```python
from build123d import *

# Parameters (mm, degrees)
F0_W     = 19.05
F0_H     = 19.05
F1_DEPTH = 19.05


with BuildPart() as f1:
    # F0 (on Front) → F1 (new body)
    with BuildSketch(Plane.XZ):
        with Locations((-9.525, 9.525)):
            Rectangle(F0_W, F0_H)
        Polygon((0, 0), (-19.05, 0), (-38.1, 0), (-38.1, -19.05), (-19.05, -19.05), (-19.05, -38.1), (0, -38.1), (0, -19.05), (19.05, -19.05), (19.05, 0), align=None)
    extrude(amount=F1_DEPTH)


solid = f1.part
```
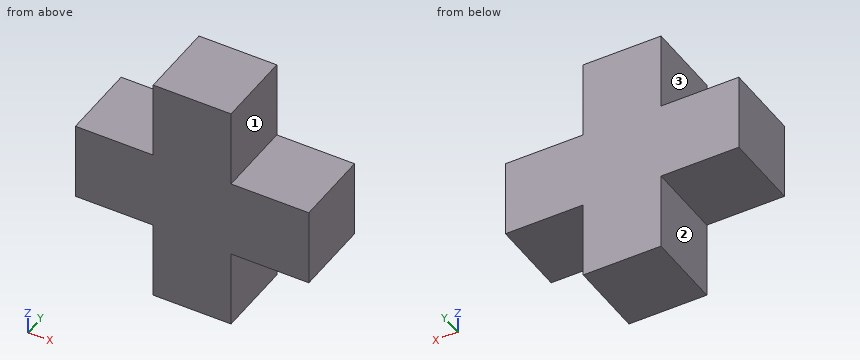
CAD build for the part. Positions are in the model's coordinates, mm. Face numbers are marked on the shaded views. A direction names the side the tool comes from. Round coordinates to 2 decimals unless told otherwise and drop trailing zeros. Write each loop counter-clockwise with the first axis right and the second up, starting at its lowest first coordinate (ties: lowest second). Pieces come first, ordered by that corner, then holes. Notation, with made-up numbers: (31, -7) - (42, -7) arc R8 cw to (42, 4) - close; hole circle Ø11 at (51.5, -22). An arc over 180 degrees is marked (long way). Write item = value, one per line. Start each with the question number.
Q1. Drop flat-ended pins along their axis: pin 1 (9.5 mm diameter, centred on y = -5, z = 12.5, fed in from +X); pin 2 (4 mm diameter, centred on x = 0.5, z = 9, fed in from -Y); pin 3 (4 mm diameter, centred on x = 12.5, y = -4, fed in from +Z); pin 4 (9.5 mm diameter, centred on y = -5.5, z = 5, fed in from -X). Give the stop position or say it passes through.
Q2. Band-saw the part on A-A (y = -8). Give the cut face in (x, z).
Q3. Probe L1, parallel to X at y = -6.75, z = 3.5. List the from-to ranges inside material, lowest first. Write a range as from..to.
Q4. Band-saw the part on B-B (x = 11). Give the cut face in (y, z), then the cut area to 3 significant figures.
Q5. Which spindle directions (+Z, -Z, +X, -X, +Y, -Y) get a long thin tool onto all of the face, cutting with end or side? Do the marked faces 1, 2 and 3. Say none if no direction does.
Answers below:
q1.pin_1 = 0
q1.pin_2 = -19.05
q1.pin_3 = 0
q1.pin_4 = -19.05
q2.outline = (-38.1, -19.05) - (-19.05, -19.05) - (-19.05, -38.1) - (0, -38.1) - (0, -19.05) - (19.05, -19.05) - (19.05, 0) - (0, 0) - (0, 19.05) - (-19.05, 19.05) - (-19.05, 0) - (-38.1, 0) - close
q3.L1 = -19.05..0
q4.outline = (-19.05, -19.05) - (0, -19.05) - (0, 0) - (-19.05, 0) - close
q4.area = 363 mm2
q5.face_1 = +Z, +X, +Y, -Y
q5.face_2 = -Z, -X, +Y, -Y
q5.face_3 = +Z, -X, +Y, -Y
